```python
from build123d import *

# Parameters (mm, degrees)
F0_R     = 11.5
F1_DEPTH = 2
F2_R     = 3.5
F3_DEPTH = 2
F4_R     = 1
F5_DEPTH = 4.001


with BuildPart() as f1:
    # F0 (on Right) → F1 (new body)
    with BuildSketch(Plane.YZ):
        Circle(F0_R)
    extrude(amount=F1_DEPTH)

    # F2 (on face) → F3 (join)
    with BuildSketch(Plane.YZ.offset(2)):
        Circle(F2_R)
    extrude(amount=F3_DEPTH)

    # F4 (on face) → F5 (cut, through all)
    with BuildSketch(Plane.YZ.offset(4)):
        Circle(F4_R)
    extrude(amount=-F5_DEPTH, mode=Mode.SUBTRACT)


solid = f1.part
```
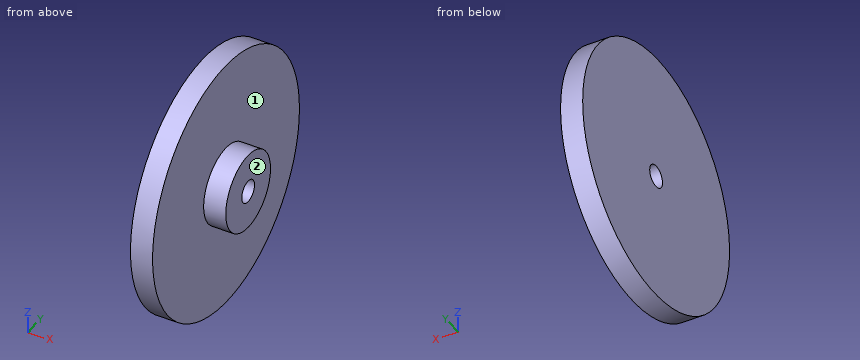
Input: part model. Units: mm. Frame: model coordinates. Face numbers are marked on the shaded views. A direction names the side the tool comes from. Coordinates: 2 decimals unless noted, no trailing zeros. Loops run counter-clockwise (first coordinate to the right, second up) from the corner with the lowest first, then second, coordinate; pieces in that order, holes last. Notation, with made-up numbers: M 18.5,-3 L 42.5,-3 A20 ccw 42.5,16 Z; hole C -36,-38 d10. An arc over 180 degrees is marked long. One line per item, written item: value.
(1) Reachability of the marked faces 1 and 2 from +Z, -Z, +X, -X, +Y, -Y: full face, straight path, thin tool, end or side. Return the list, or none.
Filled in:
face 1: +X
face 2: +Z, -Z, +X, +Y, -Y
(2) Section C-C (x = 2.3). Output: boundary loops of the cut face in (y, z).
Filled in:
outline: C 0,0 d7; hole C 0,0 d2
(3) Section D-D (z = 2.75). Output: boundary loops of the cut face in (x, y), and give its area (3 significant figures).
Filled in:
outline: M 0,-11.17 L 2,-11.17 L 2,-2.17 L 4,-2.17 L 4,2.17 L 2,2.17 L 2,11.17 L 0,11.17 Z
area: 53.3 mm^2
(4) Pin query (flat end, axial travel): pin 1 (2.5 mm diameter, centred on y = 0, z = 0, fed in from -X); pin 2 (3 mm diameter, centred on y = 6.5, z = 8.5, fed in from +X); pin 3 (1 mm diameter, centred on x = 1.5, z = -7, fed in from +Y). Return the tip coordinate at first contact, or that it passes through.
Filled in:
pin 1: x = 0
pin 2: x = 2
pin 3: y = 9.49
(5) Section A-A (y = 0). Output: boundary loops of the cut face in (x, z).
Filled in:
outline: M 0,-11.5 L 2,-11.5 L 2,-3.5 L 4,-3.5 L 4,-1 L 0,-1 Z; M 0,1 L 4,1 L 4,3.5 L 2,3.5 L 2,11.5 L 0,11.5 Z
(6) Line query: line 1 along Z through (x, y) = (2.2, 0); line 2 along Z through (x, y) = (1.45, 0); line 3 along X through (y, z) = (9.5, -4.5). Output: solid intervals per line, ascending. Write a range as from..to.
Filled in:
line 1: -3.5..-1, 1..3.5
line 2: -11.5..-1, 1..11.5
line 3: 0..2
